The figure shows three views and two pictorial views of one solid part (mm, origin at its lowest corner). Answer the questions. Coordinates: 2 decimals unless noted, no trailing zeros. Loops run counter-clockwise (first coordinate to the right, second up) from the corner with the lowest first, then second, coordinate; pieces in that order, holes last. Notation, with made-up numbers: (10, -21) -> (67, -21) arc R26 ccw to (67, -2) -> close; hole circle Ø7 at (-28.5, -33.75). An arc over 180 degrees is marked (long way). Answer as a JSON object with one key per item and string values. Group by question number.
1) Section A-A, the plane y = 10 is taken. Give the vertices of the cut face in (x, z), plus the area to 3 significant figures.
2) A flat-ended cylindrical pin translates along its axis: P1, Ø7, axis at x = 24, y = 10, coming from the +Z side. Find the tip coordinate at first contact, or state that the pin passes through.
3) Section B-B, the plane z = 1.3 is taken. Give the vertices of the cut face in (x, y), plus the area to 3 significant figures.
4) Consider probe 1 along X at (y, z) = (10, 0.4); probe 2 along Y at (x, z) = (6, 0.25); probe 3 along X at (y, z) = (11.25, 0.5). Determine where each line is inside the solid, lowest interval first. Write a range as [from, to].
5) Section C-C, the plane x = 24 is taken. Give the vertices of the cut face in (y, z).
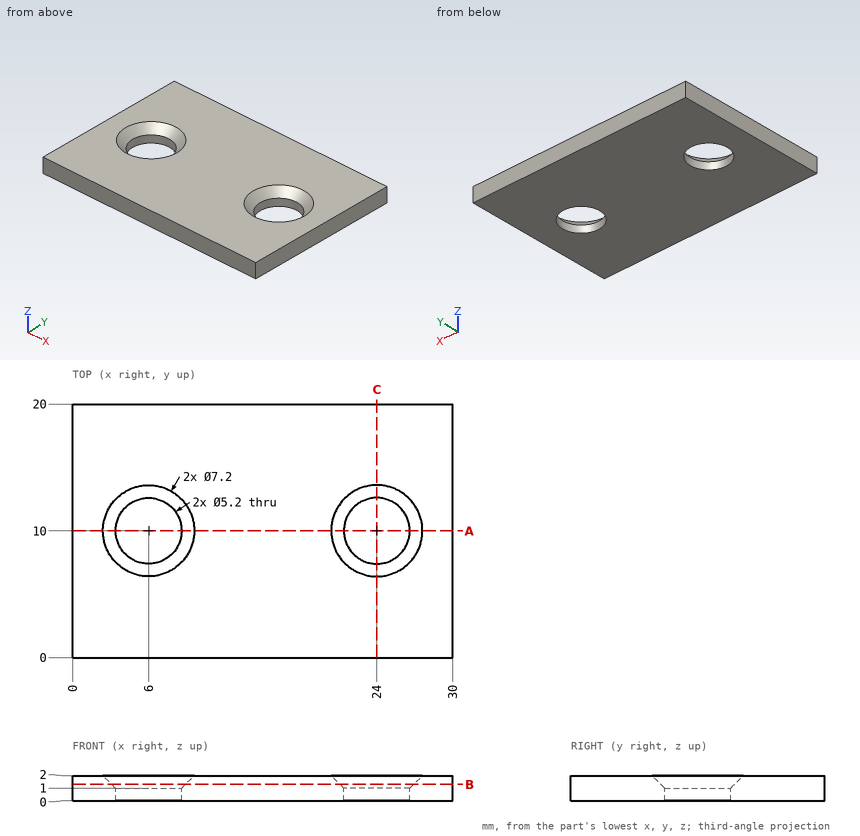
Determined:
{
 "1": {"outline": "(0, 0) -> (3.4, 0) -> (3.4, 1) -> (2.4, 2) -> (0, 2) -> close; (8.6, 0) -> (21.4, 0) -> (21.4, 1) -> (20.4, 2) -> (9.6, 2) -> (8.6, 1) -> close; (26.6, 0) -> (30, 0) -> (30, 2) -> (27.6, 2) -> (26.6, 1) -> close", "area": "37.2 mm²"},
 "2": {"P1": "z = 1.9"},
 "3": {"outline": "(0, 0) -> (30, 0) -> (30, 20) -> (0, 20) -> close; hole circle Ø5.8 at (6, 10); hole circle Ø5.8 at (24, 10)", "area": "547 mm²"},
 "4": {"probe 1": "[0, 3.4], [8.6, 21.4], [26.6, 30]", "probe 2": "[0, 7.4], [12.6, 20]", "probe 3": "[0, 3.72], [8.28, 21.72], [26.28, 30]"},
 "5": {"outline": "(0, 0) -> (7.4, 0) -> (7.4, 1) -> (6.4, 2) -> (0, 2) -> close; (12.6, 0) -> (20, 0) -> (20, 2) -> (13.6, 2) -> (12.6, 1) -> close"}
}
